The model under review builds one solid part; all positions refer to its coordinate system, in mm. A direction names the side the tool comes from. Give positions to 0.01 mm unless a question says otherwise; leave off trailing zeros. Order: outer loops, then holes, each group sorted by start corner. A loop starts at its lowest first (then second) coordinate and runs counter-clockwise, first axis right, second up. Notation, with made-up numbers: (84.25, 33.25) - (94.25, 33.25) arc R14 ccw to (94.25, 39.25) - close; hole circle Ø7 at (6.5, 27.5). An arc over 180 degrees is marked (long way). Use CSV: the item, a comma, the result in double quotes.
```python
from build123d import *

# Parameters (mm, degrees)
SKETCH_1_R          = 5.2
EXTRUDE_1_DEPTH     = 27.5
SKETCH_6_R          = 7.2
EXTRUDE_3_DEPTH     = 1.75
SKETCH_3_R          = 0.85
CUT_EXTRUDE_4_DEPTH = 8
SKETCH_7_R          = 0.9
CUT_EXTRUDE_5_DEPTH = 8


with BuildPart() as part:
    # 草图1 → 凸台-拉伸1 (new body)
    with BuildSketch(Plane.XY):
        Circle(SKETCH_1_R)
    extrude(amount=EXTRUDE_1_DEPTH)

    # 草图6 → 凸台-拉伸3 (add)
    with BuildSketch(Plane.XY.offset(27.5)):
        Circle(SKETCH_6_R)
    extrude(amount=-EXTRUDE_3_DEPTH)

    # 草图3 → 切除-拉伸4 (cut)
    with BuildSketch(Plane.XY.offset(27.5)):
        with Locations((-3, 0)):
            Circle(SKETCH_3_R)
        with Locations((3, 0)):
            Circle(SKETCH_3_R)
    cut_extrude_4 = extrude(amount=-CUT_EXTRUDE_4_DEPTH, mode=Mode.SUBTRACT)

    # 镜向3: 切除-拉伸4 across plane
    add(cut_extrude_4.mirror(Plane.XY.offset(13.75)), mode=Mode.SUBTRACT)

    # 草图7 → 切除-拉伸5 (cut)
    with BuildSketch(Plane.XY.offset(27.5)):
        with Locations((-3, 0)):
            Circle(SKETCH_7_R)
        with Locations((3, 0)):
            Circle(SKETCH_7_R)
    extrude(amount=-CUT_EXTRUDE_5_DEPTH, mode=Mode.SUBTRACT)


solid = part.part
```
Item 1: Tool access review of faces 4 (the face through (3, 0, 8)), 5 (the face through (0, 0, 27.5)), 6 (the face through (-3, 0, 19.5)): name each direction out of +Z, -Z, +X, -X, +Y, -Y from which nothing blocks a thin tool from reaching the whole face with its end or side.
Results list:
face 4,"-Z"
face 5,"+Z, +X, -X, +Y, -Y"
face 6,"+Z"
Item 2: Take a section at B-B, the plane y = 0. Give the boundary of the cut face in (x, z), and give its area (3 significant figures).
Results list:
outline,"(-7.2, 25.75) - (-5.2, 25.75) - (-5.2, 0) - (-3.85, 0) - (-3.85, 8) - (-2.15, 8) - (-2.15, 0) - (2.15, 0) - (2.15, 8) - (3.85, 8) - (3.85, 0) - (5.2, 0) - (5.2, 25.75) - (7.2, 25.75) - (7.2, 27.5) - (3.9, 27.5) - (3.9, 19.5) - (2.1, 19.5) - (2.1, 27.5) - (-2.1, 27.5) - (-2.1, 19.5) - (-3.9, 19.5) - (-3.9, 27.5) - (-7.2, 27.5) - close"
area,"237 mm2"
Item 3: Wall thickness on L1, parallel to Y at x = 3, z = 2.25; L2, parallel to Z at x = -5.5, y = 1.5; L3, parallel to Y at x = 3.5, z = 8.5: over which ranges is each line inside the solid? List them lowest first.
Results list:
L1,"y = -4.25 to -0.85, 0.85 to 4.25"
L2,"z = 25.75 to 27.5"
L3,"y = -3.85 to 3.85"
Item 4: Take a section at D-D, the plane z = 7.5. Give the boundary of the cut face in (x, y), and give its area (3 significant figures).
Results list:
outline,"circle Ø10.4 at (0, 0); hole circle Ø1.7 at (-3, 0); hole circle Ø1.7 at (3, 0)"
area,"80.4 mm2"
Item 5: Take a section at C-C, the plane z = 20.5. Give the boundary of the cut face in (x, y), and give its area (3 significant figures).
Results list:
outline,"circle Ø10.4 at (0, 0); hole circle Ø1.8 at (-3, 0); hole circle Ø1.8 at (3, 0)"
area,"79.9 mm2"
Item 6: Take a section at A-A, the plane x = 0. Give the boundary of the cut face in (y, z).
Results list:
outline,"(-7.2, 25.75) - (-5.2, 25.75) - (-5.2, 0) - (5.2, 0) - (5.2, 25.75) - (7.2, 25.75) - (7.2, 27.5) - (-7.2, 27.5) - close"
Item 7: Clearance check with flat-ended pins moving along their axes: pin 1 (0.5 mm diameter, centred on x = 3, y = 0.5, fed in from +Z); pin 2 (4 mm diameter, centred on y = -2, z = 17.5, fed in from -X); pin 3 (1.4 mm diameter, centred on x = 3, y = 0, fed in from -Z). State where each tip first meets the part, or that it passes through.
Results list:
pin 1,"stops at z = 19.5"
pin 2,"stops at x = -5.2"
pin 3,"stops at z = 8"
Item 8: Mouldability with a two-part tool opening along X and no side actions: class faces 1 (the face through (3, 0, 19.5)), 2 (the face through (0, 0, 0)), 3 (the face through (6.87, 2.16, 26.64)) as pulls with the +X half, pulls with the -X half, needs draft (parallel to the pull), parting line crosses it, or undercut.
Results list:
face 1,"undercut"
face 2,"needs draft"
face 3,"parting line crosses it"
